Design review of the part shown in the three views and the two pictorial views. Dimensions are in mm from the part's minimum x, y and z. A direction names the side the tool comes from. Give positions to 0.01 mm unless a question says otherwise; leave off trailing zeros. Order: outer loops, then holes, each group sorted by start corner. A loop starts at its lowest first (then second) coordinate and runs counter-clockwise, first axis right, second up.
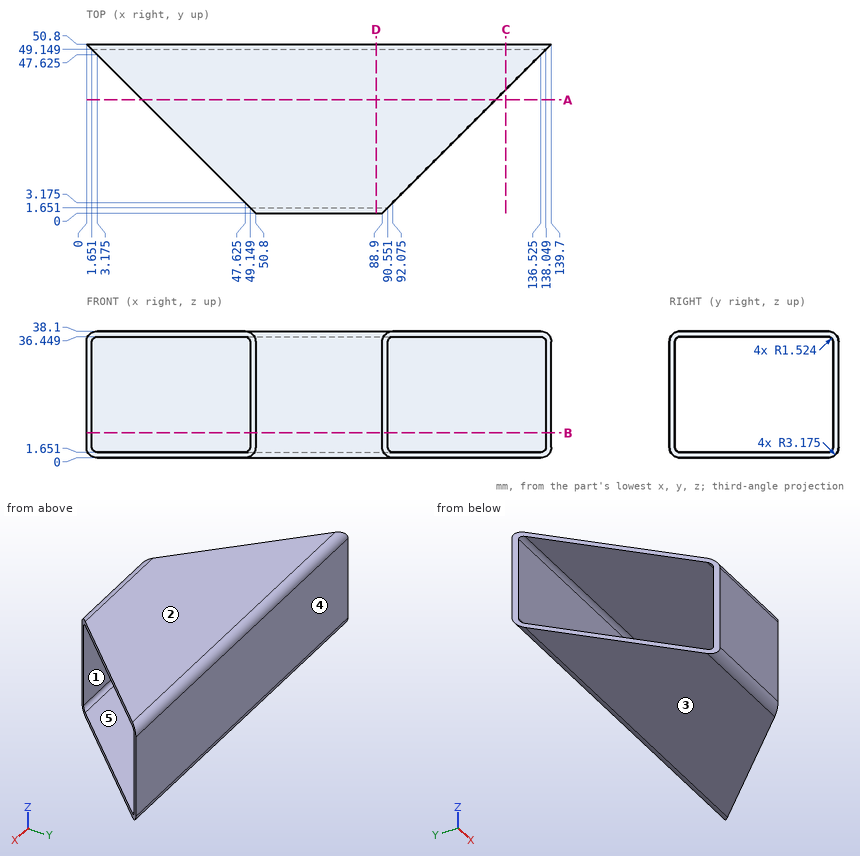
Item 1: Draft analysis for pull direction Z (two halves, no side actions). For the marked faces 3, 4 and 5, state which applies: released by +Z, released by -Z, zero draft, split by the parting line, or undercut.
Values found:
face 3: released by -Z
face 4: zero draft
face 5: undercut
Item 2: Take a section at A-A (y = 34). Give the boundary of the cut face in (x, z).
Values found:
outline: (16.8, 0) - (122.9, 0) - (122.9, 1.65) - (16.8, 1.65) - close; (16.8, 36.45) - (122.9, 36.45) - (122.9, 38.1) - (16.8, 38.1) - close
Item 3: Clearance check with a flat-ended pin moving along its axis: pin 1 Ø5 at (x, z) = (37, 29) entering from -Y. State where the tip first meets the part, or that it passes through.
Values found:
pin 1: stops at y = 49.15
Item 4: Take a section at B-B (z = 7.5). Give the boundary of the cut face in (x, y).
Values found:
outline: (0, 50.8) - (1.65, 49.15) - (138.05, 49.15) - (139.7, 50.8) - close; (49.15, 1.65) - (50.8, 0) - (88.9, 0) - (90.55, 1.65) - close
Item 5: Take a section at C-C (x = 126). Give the boundary of the cut face in (y, z) (3 decimals), and give its area (3 significant figures).
Values found:
outline: (37.1, 0) - (47.625, 0) arc R3.175 ccw to (50.8, 3.175) - (50.8, 34.925) arc R3.175 ccw to (47.625, 38.1) - (37.1, 38.1) - (37.1, 36.449) - (47.625, 36.449) arc R1.524 cw to (49.149, 34.925) - (49.149, 3.175) arc R1.524 cw to (47.625, 1.651) - (37.1, 1.651) - close
area: 99.4 mm2
Item 6: For line 1 (Z direction, x = 48, y = 18.5); line 2 (Y direction, x = 16.5, z = 21); line 3 (Y direction, x = 66.5, z = 33.5), list the stretches that pass through material, from the lowest coordinate up.
Values found:
line 1: z = 0 to 1.65, 36.45 to 38.1
line 2: y = 49.15 to 50.8
line 3: y = 0 to 1.65, 49.15 to 50.8
Item 7: For the marked faces 1 and 2, list the 3-axis set-ups (+Z, -Z, +X, -X, +Y, -Y) from which the entire face can be reached by the end or side of a thin tool; tool diameter is ignored.
Values found:
face 1: +X, -X
face 2: +Z, +X, -X, +Y, -Y
Item 8: Take a section at D-D (x = 87). Give the boundary of the cut face in (y, z) (3 decimals).
Values found:
outline: (0, 3.175) arc R3.175 ccw to (3.175, 0) - (47.625, 0) arc R3.175 ccw to (50.8, 3.175) - (50.8, 34.925) arc R3.175 ccw to (47.625, 38.1) - (3.175, 38.1) arc R3.175 ccw to (0, 34.925) - close; hole (1.651, 3.175) arc R1.524 ccw to (3.175, 1.651) - (47.625, 1.651) arc R1.524 ccw to (49.149, 3.175) - (49.149, 34.925) arc R1.524 ccw to (47.625, 36.449) - (3.175, 36.449) arc R1.524 ccw to (1.651, 34.925) - close
